CAD build for the part. Positions are in the model's coordinates, mm. Give positions to 0.01 mm unless a question says otherwise; leave off trailing zeros. Write each loop counter-clockwise with the first axis right and the second up, starting at its lowest first coordinate (ties: lowest second). Pieces come first, ordered by that corner, then holes. Notation, with made-up numbers: (89, 55.25) - (122, 55.25) arc R19 ccw to (122, 87.25) - close; hole circle Ø4 at (-35.75, 40.25). An arc over 180 degrees is marked (long way). Answer as a JSON object with one key per item and string values.
from build123d import *

# Parameters (mm, degrees)
SKETCH1_W           = 152.4
SKETCH1_H           = 88.9
SKETCH1_R           = 3.175
BOSS_EXTRUDE1_DEPTH = 2.032
CUT_EXTRUDE1_DEPTH  = 177.445739603


with BuildPart() as part:
    # Sketch1 → Boss-Extrude1 (new body)
    with BuildSketch(Plane(origin=(0, 0, 0), x_dir=(1, 0, 0), z_dir=(0, 1, 0))):
        with Locations((76.2, 44.45)):
            Rectangle(SKETCH1_W, SKETCH1_H)
        with Locations(Location((76.2, 12.7, 0), (0, 0, 270))):
            Circle(SKETCH1_R, mode=Mode.SUBTRACT)
        with Locations(Location((25.4, 12.7, 0), (0, 0, 270))):
            Circle(SKETCH1_R, mode=Mode.SUBTRACT)
        with Locations(Location((127, 12.7, 0), (0, 0, 90))):
            Circle(SKETCH1_R, mode=Mode.SUBTRACT)
    extrude(amount=BOSS_EXTRUDE1_DEPTH)

    # Sketch2 → Cut-Extrude1 (cut, through all)
    with BuildSketch(Plane.XZ):
        with BuildLine():
            ThreePointArc((141.5955, -45.174506351), (141.647276695, -44.781223305), (141.253993649, -44.833))
            ThreePointArc((141.253993649, -44.833), (141.162487298, -44.924506351), (141.037487298, -44.958))
            Line((141.037487298, -44.958), (131.362512702, -44.958))
            ThreePointArc((131.362512702, -44.958), (131.237512702, -44.924506351), (131.146006351, -44.833))
            ThreePointArc((131.146006351, -44.833), (130.752723305, -44.781223305), (130.8045, -45.174506351))
            ThreePointArc((130.8045, -45.174506351), (130.896006351, -45.266012702), (130.9295, -45.391012702))
            Line((130.9295, -45.391012702), (130.9295, -75.258987298))
            ThreePointArc((130.9295, -75.258987298), (130.896006351, -75.383987298), (130.8045, -75.475493649))
            ThreePointArc((130.8045, -75.475493649), (130.752723305, -75.868776695), (131.146006351, -75.817))
            ThreePointArc((131.146006351, -75.817), (131.237512702, -75.725493649), (131.362512702, -75.692))
            Line((131.362512702, -75.692), (141.037487298, -75.692))
            ThreePointArc((141.037487298, -75.692), (141.162487298, -75.725493649), (141.253993649, -75.817))
            ThreePointArc((141.253993649, -75.817), (141.647276695, -75.868776695), (141.5955, -75.475493649))
            ThreePointArc((141.5955, -75.475493649), (141.503993649, -75.383987298), (141.4705, -75.258987298))
            Line((141.4705, -75.258987298), (141.4705, -45.391012702))
            ThreePointArc((141.4705, -45.391012702), (141.503993649, -45.266012702), (141.5955, -45.174506351))
        make_face()
        with BuildLine():
            ThreePointArc((111.5955, -45.174506351), (111.647276695, -44.781223305), (111.253993649, -44.833))
            ThreePointArc((111.253993649, -44.833), (111.162487298, -44.924506351), (111.037487298, -44.958))
            Line((111.037487298, -44.958), (101.362512702, -44.958))
            ThreePointArc((101.362512702, -44.958), (101.237512702, -44.924506351), (101.146006351, -44.833))
            ThreePointArc((101.146006351, -44.833), (100.752723305, -44.781223305), (100.8045, -45.174506351))
            ThreePointArc((100.8045, -45.174506351), (100.896006351, -45.266012702), (100.9295, -45.391012702))
            Line((100.9295, -45.391012702), (100.9295, -75.258987298))
            ThreePointArc((100.9295, -75.258987298), (100.896006351, -75.383987298), (100.8045, -75.475493649))
            ThreePointArc((100.8045, -75.475493649), (100.752723305, -75.868776695), (101.146006351, -75.817))
            ThreePointArc((101.146006351, -75.817), (101.237512702, -75.725493649), (101.362512702, -75.692))
            Line((101.362512702, -75.692), (111.037487298, -75.692))
            ThreePointArc((111.037487298, -75.692), (111.162487298, -75.725493649), (111.253993649, -75.817))
            ThreePointArc((111.253993649, -75.817), (111.647276695, -75.868776695), (111.5955, -75.475493649))
            ThreePointArc((111.5955, -75.475493649), (111.503993649, -75.383987298), (111.4705, -75.258987298))
            Line((111.4705, -75.258987298), (111.4705, -45.391012702))
            ThreePointArc((111.4705, -45.391012702), (111.503993649, -45.266012702), (111.5955, -45.174506351))
        make_face()
        with BuildLine():
            ThreePointArc((81.5955, -45.174506351), (81.647276695, -44.781223305), (81.253993649, -44.833))
            ThreePointArc((81.253993649, -44.833), (81.162487298, -44.924506351), (81.037487298, -44.958))
            Line((81.037487298, -44.958), (71.362512702, -44.958))
            ThreePointArc((71.362512702, -44.958), (71.237512702, -44.924506351), (71.146006351, -44.833))
            ThreePointArc((71.146006351, -44.833), (70.752723305, -44.781223305), (70.8045, -45.174506351))
            ThreePointArc((70.8045, -45.174506351), (70.896006351, -45.266012702), (70.9295, -45.391012702))
            Line((70.9295, -45.391012702), (70.9295, -75.258987298))
            ThreePointArc((70.9295, -75.258987298), (70.896006351, -75.383987298), (70.8045, -75.475493649))
            ThreePointArc((70.8045, -75.475493649), (70.752723305, -75.868776695), (71.146006351, -75.817))
            ThreePointArc((71.146006351, -75.817), (71.237512702, -75.725493649), (71.362512702, -75.692))
            Line((71.362512702, -75.692), (81.037487298, -75.692))
            ThreePointArc((81.037487298, -75.692), (81.162487298, -75.725493649), (81.253993649, -75.817))
            ThreePointArc((81.253993649, -75.817), (81.647276695, -75.868776695), (81.5955, -75.475493649))
            ThreePointArc((81.5955, -75.475493649), (81.503993649, -75.383987298), (81.4705, -75.258987298))
            Line((81.4705, -75.258987298), (81.4705, -45.391012702))
            ThreePointArc((81.4705, -45.391012702), (81.503993649, -45.266012702), (81.5955, -45.174506351))
        make_face()
        with BuildLine():
            ThreePointArc((51.5955, -45.174506351), (51.647276695, -44.781223305), (51.253993649, -44.833))
            ThreePointArc((51.253993649, -44.833), (51.162487298, -44.924506351), (51.037487298, -44.958))
            Line((51.037487298, -44.958), (41.362512702, -44.958))
            ThreePointArc((41.362512702, -44.958), (41.237512702, -44.924506351), (41.146006351, -44.833))
            ThreePointArc((41.146006351, -44.833), (40.752723305, -44.781223305), (40.8045, -45.174506351))
            ThreePointArc((40.8045, -45.174506351), (40.896006351, -45.266012702), (40.9295, -45.391012702))
            Line((40.9295, -45.391012702), (40.9295, -75.258987298))
            ThreePointArc((40.9295, -75.258987298), (40.896006351, -75.383987298), (40.8045, -75.475493649))
            ThreePointArc((40.8045, -75.475493649), (40.752723305, -75.868776695), (41.146006351, -75.817))
            ThreePointArc((41.146006351, -75.817), (41.237512702, -75.725493649), (41.362512702, -75.692))
            Line((41.362512702, -75.692), (51.037487298, -75.692))
            ThreePointArc((51.037487298, -75.692), (51.162487298, -75.725493649), (51.253993649, -75.817))
            ThreePointArc((51.253993649, -75.817), (51.647276695, -75.868776695), (51.5955, -75.475493649))
            ThreePointArc((51.5955, -75.475493649), (51.503993649, -75.383987298), (51.4705, -75.258987298))
            Line((51.4705, -75.258987298), (51.4705, -45.391012702))
            ThreePointArc((51.4705, -45.391012702), (51.503993649, -45.266012702), (51.5955, -45.174506351))
        make_face()
        with BuildLine():
            ThreePointArc((21.5955, -45.174506351), (21.647276695, -44.781223305), (21.253993649, -44.833))
            ThreePointArc((21.253993649, -44.833), (21.162487298, -44.924506351), (21.037487298, -44.958))
            Line((21.037487298, -44.958), (11.362512702, -44.958))
            ThreePointArc((11.362512702, -44.958), (11.237512702, -44.924506351), (11.146006351, -44.833))
            ThreePointArc((11.146006351, -44.833), (10.752723305, -44.781223305), (10.8045, -45.174506351))
            ThreePointArc((10.8045, -45.174506351), (10.896006351, -45.266012702), (10.9295, -45.391012702))
            Line((10.9295, -45.391012702), (10.9295, -75.258987298))
            ThreePointArc((10.9295, -75.258987298), (10.896006351, -75.383987298), (10.8045, -75.475493649))
            ThreePointArc((10.8045, -75.475493649), (10.752723305, -75.868776695), (11.146006351, -75.817))
            ThreePointArc((11.146006351, -75.817), (11.237512702, -75.725493649), (11.362512702, -75.692))
            Line((11.362512702, -75.692), (21.037487298, -75.692))
            ThreePointArc((21.037487298, -75.692), (21.162487298, -75.725493649), (21.253993649, -75.817))
            ThreePointArc((21.253993649, -75.817), (21.647276695, -75.868776695), (21.5955, -75.475493649))
            ThreePointArc((21.5955, -75.475493649), (21.503993649, -75.383987298), (21.4705, -75.258987298))
            Line((21.4705, -75.258987298), (21.4705, -45.391012702))
            ThreePointArc((21.4705, -45.391012702), (21.503993649, -45.266012702), (21.5955, -45.174506351))
        make_face()
    extrude(amount=-CUT_EXTRUDE1_DEPTH, mode=Mode.SUBTRACT)


solid = part.part
(1) Flat gauge pin, fed straight in: P1, Ø0.6, axis at y = 1, z = -54.5, coming from the -X side. Where does the tip first touch, or does it go through?
Answer key:
{"P1": "stops at x = 0"}
(2) Saw through at C-C, the plane x = 76.2. Give the cut face in (y, z) (3 decimals), and give its area (3 significant figures).
Answer key:
{"outline": "(0, -88.9) - (2.032, -88.9) - (2.032, -75.692) - (0, -75.692) - close; (0, -44.958) - (2.032, -44.958) - (2.032, -15.875) - (0, -15.875) - close; (0, -9.525) - (2.032, -9.525) - (2.032, 0) - (0, 0) - close", "area": "105 mm²"}
(3) Saw through at A-A, the plane x = 127. Give the cut face in (y, z) (3 decimals).
Answer key:
{"outline": "(0, -88.9) - (2.032, -88.9) - (2.032, -15.875) - (0, -15.875) - close; (0, -9.525) - (2.032, -9.525) - (2.032, 0) - (0, 0) - close"}
(4) Saw through at B-B, the plane z = -12.7. Give the cut face in (x, y) (3 decimals), and give its area (3 significant figures).
Answer key:
{"outline": "(0, 0) - (22.225, 0) - (22.225, 2.032) - (0, 2.032) - close; (28.575, 0) - (73.025, 0) - (73.025, 2.032) - (28.575, 2.032) - close; (79.375, 0) - (123.825, 0) - (123.825, 2.032) - (79.375, 2.032) - close; (130.175, 0) - (152.4, 0) - (152.4, 2.032) - (130.175, 2.032) - close", "area": "271 mm²"}
(5) Saw through at D-D, the plane z = -48. Give the cut face in (x, y).
Answer key:
{"outline": "(0, 0) - (10.93, 0) - (10.93, 2.03) - (0, 2.03) - close; (21.47, 0) - (40.93, 0) - (40.93, 2.03) - (21.47, 2.03) - close; (51.47, 0) - (70.93, 0) - (70.93, 2.03) - (51.47, 2.03) - close; (81.47, 0) - (100.93, 0) - (100.93, 2.03) - (81.47, 2.03) - close; (111.47, 0) - (130.93, 0) - (130.93, 2.03) - (111.47, 2.03) - close; (141.47, 0) - (152.4, 0) - (152.4, 2.03) - (141.47, 2.03) - close"}
(6) Pull direction Z, two halves, no side cores. Call faces 1 (the face through (75, 0, -35)), 2 (the face through (123.85, 1, -12.29)), 3 (the face through (78.877, 1.002, -10.993)): pulls with the +Z half, pulls with the -Z half, needs draft (parallel to the pull), parting line crosses it, or undercut.
Answer key:
{"face 1": "needs draft", "face 2": "undercut", "face 3": "undercut"}
(7) Probe L1, parallel to X at y = 1.85, z = -71; L2, parallel to X at y = 0.45, z = -13; L3, parallel to Z at x = 101.5, y = 1.05. List the from-to ranges inside material, lowest first. Write a range as [from, to].
Answer key:
{"L1": "x = [0, 10.93], [21.47, 40.93], [51.47, 70.93], [81.47, 100.93], [111.47, 130.93], [141.47, 152.4]", "L2": "x = [0, 22.24], [28.56, 73.04], [79.36, 123.84], [130.16, 152.4]", "L3": "z = [-88.9, -75.69], [-44.96, 0]"}
